Check sheet for the modelled part. Datum: model origin and axes. Units: mm. A direction names the side the tool comes from. Round coordinates to 2 decimals unless told otherwise and drop trailing zeros. Loops run counter-clockwise (first coordinate to the right, second up) from the corner with the lowest first, then second, coordinate; pieces in that order, holes last. Notation, with made-up numbers: M 14.25,19 L 60.25,19 A16 ccw 60.25,45 Z; hole C -28.5,9.5 d9. An arc over 180 degrees is marked long. Write item = value, one per line. Start each with the question number.
(1) Set-up check for faces 1 (the face through (-6.571, 0, 244)), 2 (the face through (5, -13, 227.584)), 3 (the face through (1, 10.165, 244)), 4 (the face through (28, -28, 156.464)): record each of +Z, -Z, +X, -X, +Y, -Y from which the full face is reachable in a straight line by a thin tool's end or side.
(2) Cross-section at A-A on z = 59.5. Record the boundary of the cut face in (x, y).
(3) Scan lines: L1, parallel to X at y = 1.5, z = 87; L2, parallel to Y at x = 1, z = 94; L3, parallel to Z at x = -39, y = 2.5. Record each from-to range of solid material in increasing order. Write a range as from..to.
(4) Go/stop test with flat-tipped pins: P1, Ø12, axis at x = -1, z = 240, coming from the -Y side; P2, Ø2, axis at x = 28.5, z = 102.5, coming from the -Y side; P3, Ø10, axis at x = 2.5, z = 202, coming from the +Y side. Record where each tip stops, or that it passes through.
(5) Cross-section at B-B on z = 23. Record the boundary of the cut face in (x, y).
from build123d import *

# Parameters (mm, degrees)
F0_R        = 50.8095284436
F1_DEPTH    = 19.05
F2_R        = 4.318
F3_R        = 2.54
F5_R        = 38.1
F6_DEPTH    = 137.414
F8_R        = 64.7161809078
F1_FACE_R   = 46.4915284436
F1_FACE_R_2 = 38.1
F9_DEPTH    = 15.494
F11_R       = 54.8295431731
F12_DEPTH   = 39.624
F13_R       = 34.3397737112
F15_R       = 26.8787144504
F16_DEPTH   = 16.002
F17_R       = 12.7
F19_R       = 13.3764834425
F20_DEPTH   = 7.62
F22_W       = 15.0005891919
F22_H       = 19.6202434599
F23_DEPTH   = 17.78


with BuildPart() as f1:
    # F0 (on Top) → F1 (new body)
    with BuildSketch(Plane.XY):
        Circle(F0_R)
    extrude(amount=F1_DEPTH)

    # F2
    f2_edges = [f1.edges().sort_by_distance(p)[0] for p in [
        (-50.809528, 0, 19.05),
    ]]
    fillet(f2_edges, radius=F2_R)

    # F3
    f3_edges = [f1.edges().sort_by_distance(p)[0] for p in [
        (-50.809528, 0, 0),
    ]]
    fillet(f3_edges, radius=F3_R)

    # F5 (on offset) → F6 (join)
    with BuildSketch(Plane.XY.offset(19.05)):
        Circle(F5_R)
    extrude(amount=F6_DEPTH)

    # F8 (on offset) + F1_face (on face) → F9 (join)
    with BuildSketch(Plane.XY.offset(156.464)):
        Circle(F8_R)
    with BuildSketch(Plane.XY.offset(19.05)):
        Circle(F1_FACE_R)
        Circle(F1_FACE_R_2, mode=Mode.SUBTRACT)
    extrude(amount=F9_DEPTH)

    # F11 (on offset) → F12 (join)
    with BuildSketch(Plane.XY.offset(171.958)):
        Circle(F11_R)
    extrude(amount=F12_DEPTH)

    # F13
    f13_edges = [f1.edges().sort_by_distance(p)[0] for p in [
        (-54.829543, 0, 211.582),
    ]]
    fillet(f13_edges, radius=F13_R)

    # F15 (on offset) → F16 (join)
    with BuildSketch(Plane.XY.offset(211.582)):
        Circle(F15_R)
    extrude(amount=F16_DEPTH)

    # F17
    f17_edges = [f1.edges().sort_by_distance(p)[0] for p in [
        (-26.878714, 0, 227.584),
    ]]
    fillet(f17_edges, radius=F17_R)

    # F19 (on offset) → F20 (join)
    with BuildSketch(Plane.XY.offset(227.584)):
        Circle(F19_R)
    extrude(amount=F20_DEPTH)

    # F22 (on offset) → F23 (join)
    with BuildSketch(Plane.XY.offset(235.204)):
        with Locations((0.9291712195, 0.3550583497)):
            Rectangle(F22_W, F22_H)
    extrude(amount=F23_DEPTH)


solid = f1.part
Result:
q1.face_1 = +Z, -X, +Y, -Y
q1.face_2 = +Z
q1.face_3 = +Z, +X, -X, +Y
q1.face_4 = none
q2.outline = C 0,0 d76.2
q3.L1 = -38.07..38.07
q3.L2 = -38.09..38.09
q3.L3 = 0..34.54, 156.46..206.11
q4.P1 = -13.38
q4.P2 = -26.37
q4.P3 = 48.52
q5.outline = C 0,0 d92.98
